Autodesk Inventor part; units mm, degrees
ref_plane "Work Plane1" through (6, 0, 0) normal (-1, 0, 0) x (0, 0, -1)
ref_plane "Work Plane2" through (0, 15, 0) normal (0, 1, 0) x (-1, 0, 0)
ref_plane "YZ Plane" through (0, 0, 0) normal (1, 0, 0) x (0, 1, 0)
sketch "Sketch1" plane through (0, 0, 0) normal (0, 1, 0) x (-1, 0, 0)
  line L0 (0, 0) -> (0, 35.75)
  line L1 (0, 0) -> (-56, 0)
  line L2 (-56, 0) -> (-56, 33.9625)
  line L3 (11.2, 0) -> (-67.2, 0)
  line L4 (-50, 30.1718) -> (-50, 6)
  line L5 (-6, 6) -> (-6, 30.7506)
  line L6 (-6, 30.7506) -> (-50, 30.1718)
  line L7 (-28, 0) -> (-28, 30.4612)
  line L8 (-16, 0) -> (-16, 30.619)
  line L9 (-40, 0) -> (-40, 30.3033)
  line L10 (-50, 6) -> (-40, 6)
  line L11 (-16, 6) -> (-6, 6)
  line L12 (0, 35.75) -> (-12, 35.75)
  line L13 (-12, 35.75) -> (-56, 33.9625)
  dimension "d1" = 33.9625
  dimension "d8" = 35.75
  dimension "d10" = 56
  dimension "d22" = 28
  dimension "d23" = 12
  dimension "d24" = 12
  dimension "d29" = 12
revolve "Revolution1" add sketch "Sketch1" angle 180 about axis through (-10, 0, 0) along (-1, 0, 0) contours L1 L8 L11 L5 L6 L4 L10 L9 L2 L13 L12 L0 | L1 L7 L6 L8 | L1 L9 L6 L7
ref_plane "Work Plane1" through (6, 0, 0) normal (-1, 0, 0) x (0, 0, -1)
sketch "Sketch3" plane through (6, 0, 0) normal (-1, 0, 0) x (0, 0, -1)
  line L0 (-15, 15) -> (15, 15)
  line L1 (15, 15) -> (15, -15)
  line L2 (15, -15) -> (-15, -15)
  line L3 (-15, -15) -> (-15, 15)
  line L4 (-15, 15) -> (15, -15) construction
  line L5 (15, 15) -> (-15, -15) construction
  point P0 (0, 0)
  dimension "d12" = 30
  dimension "d13" = 30
extrude "Extrusion2" cut sketch "Sketch3" against normal blind 44
sketch "Sketch4" plane through (0, 0, 0) normal (-1, 0, 0) x (0, 0, -1)
  circle A0 centre (0, 0) radius 14.5
  point P0 (0, 0)
  dimension "d16" = 29
extrude "Extrusion3" cut sketch "Sketch4" against normal blind 6
sketch "Sketch5" plane through (56, 0, 0) normal (1, 0, 0) x (0, 0, -1)
  line L0 (14.25, -14.25) -> (-14.25, -14.25)
  line L1 (-14.25, -14.25) -> (-14.25, 14.25)
  line L2 (-14.25, 14.25) -> (14.25, 14.25)
  line L3 (14.25, 14.25) -> (14.25, -14.25)
  line L4 (14.25, -14.25) -> (-14.25, 14.25) construction
  line L5 (-14.25, -14.25) -> (14.25, 14.25) construction
  point P0 (0, 0)
  dimension "d25" = 28.5
  dimension "d26" = 28.5
extrude "Extrusion4" cut sketch "Sketch5" against normal blind 6
chamfer "Chamfer3" distance 1 angle 45 1 edges at (0, 35.75, 0)
sketch "Sketch6" plane through (16, 0, 15) normal (0, -1, 0) x (1, 0, 0)
  line L0 (-16, 19.75) -> (-15, 20.75)
  line L1 (-16, -0.5) -> (-16, 19.75)
  line L2 (-16, -0.5) -> (-10, -0.5)
  line L3 (-10, -0.5) -> (-10, 15.7506)
  line L4 (-10, 15.7506) -> (0, 15.619)
  line L5 (0, 15.619) -> (0, 0)
  line L6 (0, 0) -> (24, 0)
  line L7 (24, 0) -> (24, 15.3033)
  line L8 (24, 15.3033) -> (34, 15.1718)
  line L9 (34, 15.1718) -> (34, -0.75)
  line L10 (34, -0.75) -> (40, -0.75)
  line L11 (40, 18.9625) -> (40, -0.75)
  line L12 (-4, 20.75) -> (40, 18.9625)
  line L13 (-15, 20.75) -> (-4, 20.75)
  line L14 (-16, -15) -> (40, -15)
  line L15 (40, -0.75) -> (40, -29.25)
  line L16 (13, -15) -> (38, -15) construction
  line L17 (12, -15) -> (12, 10)
  line L18 (12, -15) -> (37, -15) construction
  circle A0 centre (12, 10) radius 1.5
  dimension "d46" = 25
  dimension "d47" = 90
  dimension "d48" = 3
extrude "Extrusion5" cut sketch "Sketch6" against normal through all contours A0
ref_plane "Work Plane2" through (0, 15, 0) normal (0, 1, 0) x (-1, 0, 0)
sketch "Sketch7" plane through (0, 15, 0) normal (0, 1, 0) x (-1, 0, 0)
  circle A0 centre (-28, 25) radius 1.5
  arc A1 (-35.5, 25) -> (-20.5, 25) centre (-28, 25) ccw
  spline S0 degree 5 poles (-29.5, 25) (-29.5, 25.2111) (-29.4629, 25.4204) (-29.3897, 25.6231) (-29.2804, 25.8128) (-29.0332, 26.0983) (-28.9152, 26.2048) (-28.7791, 26.2979) (-28.6269, 26.3735) (-28.3307, 26.4697) (-28.1905, 26.4982) (-28.0469, 26.5095) (-27.9041, 26.5034) (-27.5429, 26.4465) (-27.3324, 26.3699) (-27.1499, 26.2607) (-26.9942, 26.1299) (-26.7049, 25.7958) (-26.5873, 25.5835) (-26.513, 25.3527) (-26.4842, 25.1114) (-26.5242, 24.6611) (-26.578, 24.4533) (-26.6719, 24.2502) (-26.8064, 24.0618) (-27.1556, 23.7366) (-27.3724, 23.6017) (-27.6224, 23.5132) (-27.8827, 23.4833) (-28.3338, 23.524) (-28.5277, 23.5752) (-28.7076, 23.6563) (-28.8674, 23.7623) (-29.2025, 24.0647) (-29.3531, 24.2808) (-29.4523, 24.5167) (-29.5, 24.7592) (-29.5, 25) knots 0 0 0 0 0 0 0.12181 0.12181 0.12181 0.12181 0.205743 0.205743 0.205743 0.205743 0.273981 0.273981 0.273981 0.273981 0.384852 0.384852 0.384852 0.384852 0.524069 0.524069 0.524069 0.524069 0.641928 0.641928 0.641928 0.641928 0.764397 0.764397 0.764397 0.764397 0.86105 0.86105 0.86105 0.86105 1 1 1 1 1 1
  line L0 (-12, 35.75) -> (-56, 33.9625)
  line L1 (-56, 33.9625) -> (-56, -33.9625)
  line L2 (-12, -35.75) -> (-56, -33.9625)
  line L3 (-12, 35.75) -> (-12, -35.75)
  line L4 (-20.5, 25) -> (-20.5, 35.4047)
  line L5 (-35.5, 25) -> (-35.5, 34.7953)
  point P0 (0, 0)
  dimension "d50" = 15
extrude "Extrusion7" cut sketch "Sketch7" along normal blind 40 contours L5 L0 L4 A1
sketch "Sketch8" plane through (0, 0, 0) normal (-1, 0, 0) x (0, 0, 1)
  line L0 (0, 0) -> (0, 19.5)
  line L1 (0, 19.5) -> (15, 19.5)
  line L2 (15, 19.5) -> (15, 29.5)
  line L3 (15, 29.5) -> (-15, 29.5)
  line L4 (-15, 29.5) -> (-15, 19.5)
  line L5 (-15, 19.5) -> (0, 19.5)
  dimension "d61" = 19.5
  dimension "d62" = 15
  dimension "d63" = 10
  dimension "d64" = 30
  dimension "d65" = 90
  dimension "d66" = 10
extrude "Extrusion8" cut sketch "Sketch8" against normal blind 3
mirror "Mirror3" about plane through (0, 0, 0) normal (0, 0, 1) of "Extrusion5", "Extrusion7"
sketch "Sketch10" plane through (3, 0, 0) normal (-1, 0, 0) x (0, 0, 1)
  line L0 (15, 19.5) -> (-15, 19.5)
  line L1 (15, 29.5) -> (15, 19.5)
  line L2 (-15, 29.5) -> (15, 29.5)
  line L3 (-15, 19.5) -> (-15, 29.5)
  line L4 (-15, 19.5) -> (-15, 29.5)
  line L5 (-15, 19.5) -> (15, 29.5)
  circle A0 centre (0, 24.5) radius 2.5
  point P0 (0, 0)
  dimension "d67" = 5
extrude "Extrusion9" cut sketch "Sketch10" against normal up to next contours A0 L5 | L5 A0
equation "\"d8\" = 0.5 * pipeID"
equation "\"d22\" = 0.5 * d10"
equation "\"d23\" = 2 * wallTh"
equation "\"d24\" = 2 * wallTh"
equation "\"d29\" = 2 * wallTh"
equation "\"d17\" = wallTh"
equation "\"d27\" = wallTh"
equation "\"pipeID\" = 71.5"
equation "\"wallTh\" = 6"
equation "\"taper\" = 0.95"
equation "\"d11\" = -wallTh"
properties part number "cameraHolder"
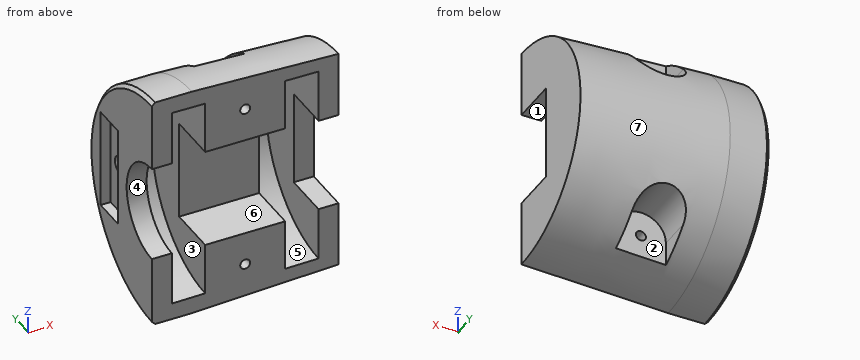
Model file for the job. Use its own axes, mm. Face numbers are marked on the shaded views. A direction names the side the tool comes from. Give positions to 0.01 mm unless a question says otherwise; leave off trailing zeros. Order: outer loops, then holes, each group sorted by start corner. A loop starts at its lowest first (then second) coordinate and runs counter-clockwise, first axis right, second up. Notation, with made-up numbers: M -18.75,-29.75 L -3.75,-29.75 A26 ccw -3.75,-14.75 Z; hole C 6,77.5 d1. An arc over 180 degrees is marked long. Put each result on its own line as item: value. Start each with the question number.
(1) Tool access for the marked faces 1, 2 and 3: list every direction of +Z, -Z, +X, -X, +Y, -Y with a clear straight run to the whole face (end or side of a thin tool).
(2) Pull direction X, two halves, no side cores. Call the marked faces 4, 5, 6 and 7: released by +X, released by -X, zero draft, split by the parting line, or undercut.
(3) Pin check, flat tips, straight feed: pin 1 Ø1.5 at (x, y) = (12.5, 8.5) entering from +Z; pin 2 Ø1 at (x, y) = (42.5, 27) entering from -Z; pin 3 Ø5 at (x, z) = (28, -25) entering from -Y; pin 4 Ø1.5 at (x, z) = (1, 3) entering from +Y. Stop position of each tip, or through.
(4) Band-saw the part on B-B on y = 7.5. Count the separate pieces of the cut face and the enclosed holes in it, then the cut area to 3 significant figures.
(5) Band-saw the part on A-A on x = 28. Give the cut face in (y, z).
(6) Drill centre lines: L1, parallel to X at y = 11, z = -25; L2, parallel to X at y = 26, z = 7.5; L3, parallel to X at y = 20, z = -16.5. Where is each one in solid material? Low to high. Write a range as [from, to].
Results below:
1. face 1: +X, -Y
1. face 2: -Z, +Y
1. face 3: -Y
2. face 4: zero draft
2. face 5: undercut
2. face 6: undercut
2. face 7: released by +X
3. pin 1: stops at z = 34.88
3. pin 2: stops at z = -22.11
3. pin 3: stops at y = 0
3. pin 4: stops at y = 35.68
4. separate pieces: 2
4. enclosed holes: 2
4. area: 1,600 mm2
5. outline: M 0,-35.1 A35.1 ccw 15,-31.73 L 15,-26.5 L 0,-26.5 Z; M 0,-23.5 L 15,-23.5 L 15,-17.5 L 30.43,-17.5 A35.1 ccw 30.43,17.5 L 15,17.5 L 15,23.5 L 0,23.5 L 0,15 L 15,15 L 15,-15 L 0,-15 Z; M 0,26.5 L 15,26.5 L 15,31.73 A35.1 ccw 0,35.1 Z
6. L1: x = [0, 6], [16, 26.5], [29.5, 40], [50, 56]
6. L2: x = [3, 6], [16, 40], [50, 56]
6. L3: x = [0, 6], [16, 40], [50, 56]
